Read the model definition and answer for the solid it produces. Units are mm, in the model's axes. Face numbers are marked on the shaded views. A direction names the side the tool comes from. Coordinates: 2 decimals unless noted, no trailing zeros. Write each loop counter-clockwise with the first axis right and the second up, starting at its lowest first coordinate (ties: lowest second). Pieces come first, ordered by that corner, then holes. Notation, with made-up numbers: M -31,32.25 L 4,32.25 A11 ccw 4,36.25 Z; hole C 1.5,-1.5 d1. An arc over 180 degrees is marked long. Write item = value, one per line.
from build123d import *

# Parameters (mm, degrees)
F3_DEPTH = 3
F4_DEPTH = 3
F0_W     = 1
F0_H     = 3
F5_DEPTH = 125
F7_DEPTH = 3


with BuildPart() as f3:
    # F1 (on Top) → F3 (new body)
    with BuildSketch(Plane.XY):
        Polygon((-19, 0), (-2.7684667148, 0), (-2.7684667148, 125), (-19, 125), (-19, 102), (-19, 23), align=None)
        with BuildLine():
            ThreePointArc((-8.95, 23), (-10.7, 21.25), (-12.45, 23))
            ThreePointArc((-12.45, 23), (-10.7, 24.75), (-8.95, 23))
        make_face(mode=Mode.SUBTRACT)
        with BuildLine():
            ThreePointArc((-8.95, 102), (-10.7, 100.25), (-12.45, 102))
            ThreePointArc((-12.45, 102), (-10.7, 103.75), (-8.95, 102))
        make_face(mode=Mode.SUBTRACT)
    extrude(amount=F3_DEPTH)

    # F2 (on Right) → F4 (join)
    with BuildSketch(Plane.YZ):
        Polygon((0, 3), (0, 0), (0, -17), (125, -17), (125, 3), align=None)
    extrude(amount=-F4_DEPTH)

    # F0 (on Front) → F5 (join)
    with BuildSketch(Plane.XZ):
        with Locations((0.5, -15.5)):
            Rectangle(F0_W, F0_H)
    extrude(amount=-F5_DEPTH)

    # F6 (on face) → F7 (join)
    with BuildSketch(Plane.XY.offset(-14)):
        with BuildLine():
            Line((1, 125), (1, 0))
            Line((1, 0), (5.2, 0))
            Line((5.2, 0), (5.2, 28.45))
            ThreePointArc((5.2, 28.45), (3.45, 30.2), (5.2, 31.95))
            Line((5.2, 31.95), (5.2, 48.45))
            ThreePointArc((5.2, 48.45), (3.45, 50.2), (5.2, 51.95))
            Line((5.2, 51.95), (5.2, 73.05))
            ThreePointArc((5.2, 73.05), (3.45, 74.8), (5.2, 76.55))
            Line((5.2, 76.55), (5.2, 93.05))
            ThreePointArc((5.2, 93.05), (3.45, 94.8), (5.2, 96.55))
            Line((5.2, 96.55), (5.2, 125))
            Line((5.2, 125), (1, 125))
        make_face()
        with BuildLine():
            Line((5.2, 28.45), (5.2, 0))
            Line((5.2, 0), (10, 0))
            Line((10, 0), (10, 125))
            Line((10, 125), (6.2, 125))
            Line((6.2, 125), (5.2, 125))
            Line((5.2, 125), (5.2, 96.55))
            ThreePointArc((5.2, 96.55), (6.4374368671, 96.0374368671), (6.95, 94.8))
            ThreePointArc((6.95, 94.8), (6.4374368671, 93.5625631329), (5.2, 93.05))
            Line((5.2, 93.05), (5.2, 76.55))
            ThreePointArc((5.2, 76.55), (6.4374368671, 76.0374368671), (6.95, 74.8))
            ThreePointArc((6.95, 74.8), (6.4374368671, 73.5625631329), (5.2, 73.05))
            Line((5.2, 73.05), (5.2, 51.95))
            ThreePointArc((5.2, 51.95), (6.4374368671, 51.4374368671), (6.95, 50.2))
            ThreePointArc((6.95, 50.2), (6.4374368671, 48.9625631329), (5.2, 48.45))
            Line((5.2, 48.45), (5.2, 31.95))
            ThreePointArc((5.2, 31.95), (6.4374368671, 31.4374368671), (6.95, 30.2))
            ThreePointArc((6.95, 30.2), (6.4374368671, 28.9625631329), (5.2, 28.45))
        make_face()
    extrude(amount=-F7_DEPTH)


solid = f3.part
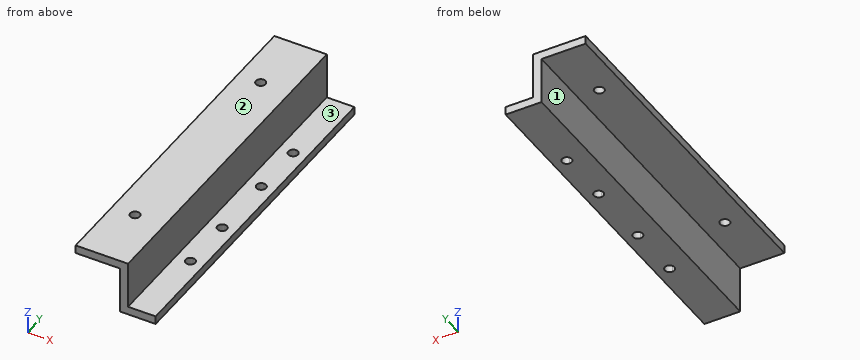
Item 1: Find section A-A (y = 23). Determine the outline of the cut face in (x, z).
Worked answers:
outline = M -19,0 L -12.45,0 L -12.45,3 L -19,3 Z; M -8.95,0 L -3,0 L -3,-17 L 10,-17 L 10,-14 L 0,-14 L 0,3 L -8.95,3 Z
Item 2: Find section B-B (x = -10.7). Determine the outline of the cut face in (y, z).
Worked answers:
outline = M 0,0 L 21.25,0 L 21.25,3 L 0,3 Z; M 24.75,0 L 100.25,0 L 100.25,3 L 24.75,3 Z; M 103.75,0 L 125,0 L 125,3 L 103.75,3 Z
Item 3: Consider line 1 along Y through (x, z) = (-10.7, 0.6); line 2 along X through (y, z) = (117, -14.5); line 3 along Z through (x, y) = (1.25, 12.5). Determine where each line is inside the solid, lowest interval first. Write a range as from..to.
Worked answers:
line_1 = 0..21.25, 24.75..100.25, 103.75..125
line_2 = -3..10
line_3 = -17..-14
Item 4: Which of the six approach directions +Z, -Z, +X, -X, +Y, -Y give full straight-line access (tool end or side, diameter ignored) to the marked faces 1, 2 and 3?
Worked answers:
face_1 = -Z, -X, +Y, -Y
face_2 = +Z, +X, -X, +Y, -Y
face_3 = +Z, +X, +Y, -Y
Item 5: Flat-ended cylindrical pins translate along their axes: pin 1 (3 mm diameter, centred on x = 2.5, y = 57, fed in from +Z); pin 2 (5 mm diameter, centred on x = -7, y = 98, fed in from -Z); pin 3 (6 mm diameter, centred on y = 77, z = -4.5, fed in from +X); pin 4 (4 mm diameter, centred on x = 2.5, z = -10.5, fed in from -Y). Find the tip coordinate at first contact, or state that the pin passes through.
Worked answers:
pin_1 = -14
pin_2 = 0
pin_3 = 0
pin_4 = through
Item 6: Find section C-C (z = -10.5). Determine the outline of the cut face in (x, y).
Worked answers:
outline = M -3,0 L 0,0 L 0,125 L -3,125 Z
